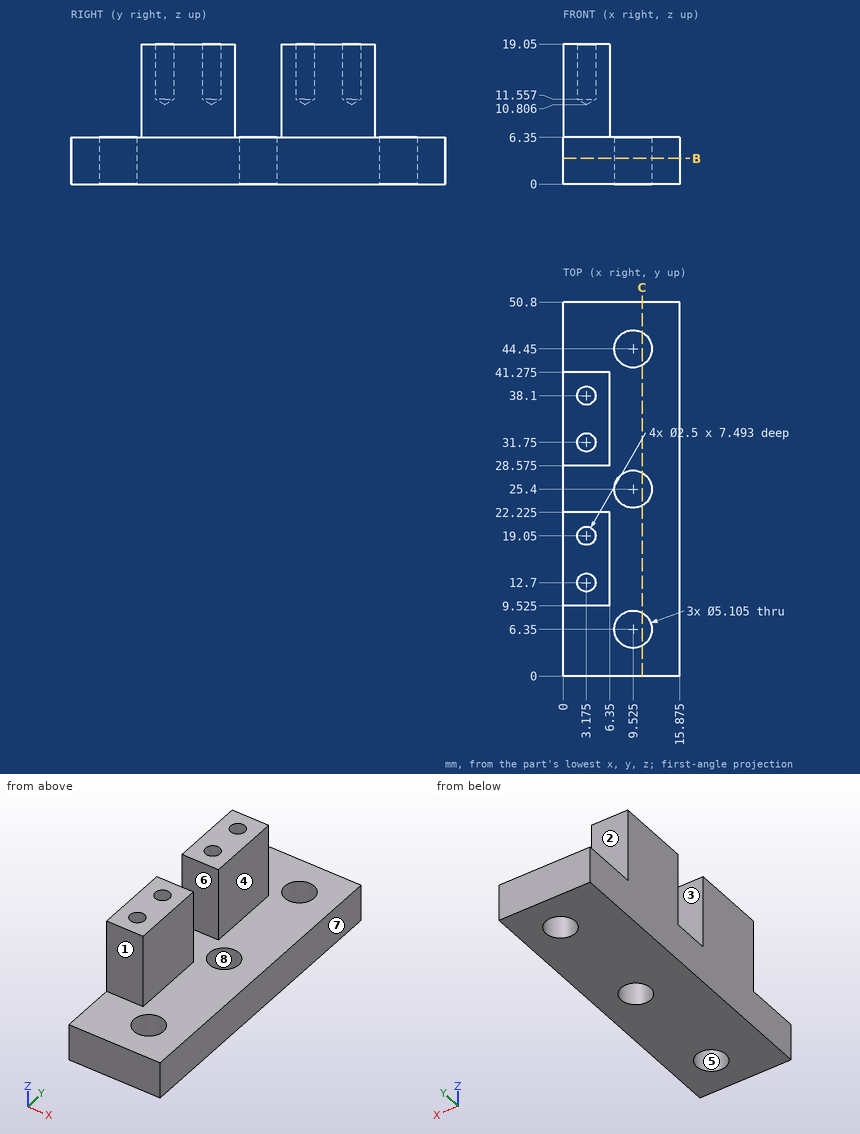
The figure shows three views and two pictorial views of one solid part (mm, origin at its lowest corner). Answer the questions. A direction names the side the tool comes from. Give positions to 0.01 mm unless a question says otherwise; leave off trailing zeros. Order: outer loops, then holes, each group sorted by start corner. A loop starts at its lowest first (then second) coordinate and runs counter-clockwise, first axis right, second up. Notation, with made-up numbers: M -13.75,49 L 40.25,49 A8 cw 40.25,56 Z; hole C -4,82.5 d4. An arc over 180 degrees is marked long. Return JSON: item names as keys, results as strings.
Q1. Find section C-C, the plane x = 10.75. Write down the section's boundary in (y, z).
Answer below:
{"outline": "M 0,0 L 4.11,0 L 4.11,6.35 L 0,6.35 Z; M 8.59,0 L 23.16,0 L 23.16,6.35 L 8.59,6.35 Z; M 27.64,0 L 42.21,0 L 42.21,6.35 L 27.64,6.35 Z; M 46.69,0 L 50.8,0 L 50.8,6.35 L 46.69,6.35 Z"}
Q2. The mould has two halves that part along X. Classify the marked faces 5, 6, 7 and 8: pulls with the +X half, pulls with the -X half, needs draft (parallel to the pull), parting line crosses it, or undercut.
Answer below:
{"face 5": "undercut", "face 6": "needs draft", "face 7": "pulls with the +X half", "face 8": "undercut"}
Q3. Find the intervals of material crossed by line 1 along Y through (x, z) = (1.75, 8.25) (1 decimal); line 2 along Z through (x, y) = (11.5, 46.5); line 3 along Y through (x, z) = (8.5, 1), in increasing order. Write a range as [from, to].
Answer below:
{"line 1": "y = [9.5, 22.2], [28.6, 41.3]", "line 2": "z = [0, 6.35]", "line 3": "y = [0, 4.01], [8.69, 23.06], [27.74, 42.11], [46.79, 50.8]"}
Q4. Find section B-B, the plane z = 3.5. State how many separate pieces and enclosed holes the cut face has, and give its area (3 significant figures).
Answer below:
{"separate pieces": "1", "enclosed holes": "3", "area": "745 mm^2"}
Q5. Each of these flat-tipped pins is pushed along its axis until it touches: pin 1 (7 mm diameter, centred on x = 4.5, z = 11.5, fed in from +Y) (3 decimals); pin 2 (6.5 mm diameter, centred on y = 32, z = 13, fed in from +X); pin 3 (3 mm diameter, centred on x = 3.5, z = 13.5, fed in from -Y) (3 decimals); pin 4 (3 mm diameter, centred on x = 9.525, y = 25.4, fed in from -Z) (3 decimals). Where does it stop, or does it pass through?
Answer below:
{"pin 1": "stops at y = 41.275", "pin 2": "stops at x = 6.35", "pin 3": "stops at y = 9.525", "pin 4": "passes through"}
Q6. Which of the six approach directions +Z, -Z, +X, -X, +Y, -Y give full straight-line access (tool end or side, diameter ignored) to the marked faces 1, 2, 3 and 4?
Answer below:
{"face 1": "+Z, +X, -X, -Y", "face 2": "+Z, +X, -X, +Y", "face 3": "+Z, +X, -X", "face 4": "+Z, +X, +Y, -Y"}
